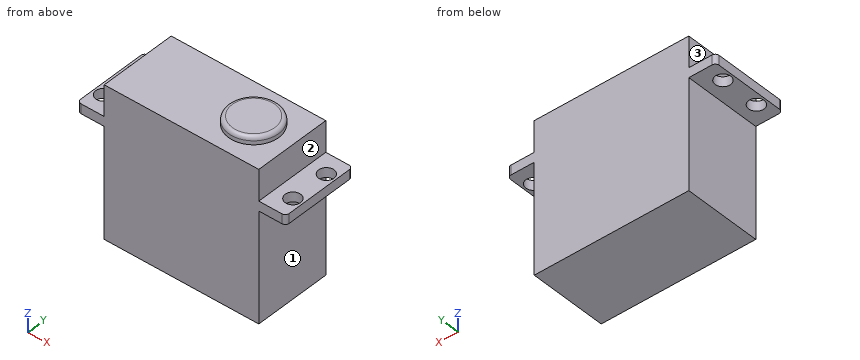
from build123d import *

# Parameters (mm, degrees)
PAD050_DEPTH    = 10
SKETCH087_R     = 2
POCKET033_DEPTH = 47.001
FILLET024_R     = 1
SKETCH235_R     = 6.5
PAD096_DEPTH    = 2
FILLET011_R     = 1


with BuildPart() as part:
    # Sketch086 → Pad050 (new body, symmetric)
    with BuildSketch(Plane.XZ):
        Polygon((-37, -18.5), (-37, -16), (-30, -16), (-30, -8), (10, -8), (10, -16), (17, -16), (17, -18.5), (10, -18.5), (10, -47), (-30, -47), (-30, -18.5), align=None)
    extrude(amount=PAD050_DEPTH, both=True)

    # Sketch087 → Pocket033 (cut, through all)
    with BuildSketch(Plane.XY):
        with Locations((14.5, 5)):
            Circle(SKETCH087_R)
        with Locations((14.5, -5)):
            Circle(SKETCH087_R)
        with Locations((-34.5, 5)):
            Circle(SKETCH087_R)
        with Locations((-34.5, -5)):
            Circle(SKETCH087_R)
    extrude(amount=-POCKET033_DEPTH, mode=Mode.SUBTRACT)

    # Fillet024
    fillet024_edges = [part.edges().sort_by_distance(p)[0] for p in [
        (17, -10, -17.25),
        (17, 10, -17.25),
        (-37, -10, -17.25),
        (-37, 10, -17.25),
    ]]
    fillet(fillet024_edges, radius=FILLET024_R)

    # Sketch235 (on Face12 of Fillet024) → Pad096 (join)
    with BuildSketch(Plane(origin=(0, 0, -8), x_dir=(-1, 0, 0), z_dir=(0, 0, 1))):
        Circle(SKETCH235_R)
    extrude(amount=PAD096_DEPTH)

    # Fillet011
    fillet011_edges = [part.edges().sort_by_distance(p)[0] for p in [
        (6.5, 0, -6),
    ]]
    fillet(fillet011_edges, radius=FILLET011_R)


with BuildPart() as part_1:
    # Body041 placement: moved
    add(part.part.moved(Location((0, 0, -1))))


solid = part_1.part
Part model, mm, in its own coordinate system. Face numbers are marked on the shaded views. A direction names the side the tool comes from. Coordinates: 2 decimals unless noted, no trailing zeros. Write each loop counter-clockwise with the first axis right and the second up, starting at its lowest first coordinate (ties: lowest second). Pieces come first, ordered by that corner, then holes. Notation, with made-up numbers: M 18,-32.5 L 54,-32.5 A24 cw 54,-8.5 Z; hole C 15.5,23 d9. An arc over 180 degrees is marked long. Return JSON: item names as keys, results as strings.
1. Flat gauge pins, fed straight in: pin 1 Ø7.5 at (x, y) = (-34.5, 0.5) entering from +Z; pin 2 Ø1 at (y, z) = (-7, -26) entering from +X; pin 3 Ø4 at (y, z) = (0.5, -11) entering from -X; pin 4 Ø2.5 at (x, y) = (-34.5, 5) entering from +Z. Where does each tip first touch, or does it go through?
Determined:
{"pin 1": "z = -17", "pin 2": "x = 10", "pin 3": "x = -30", "pin 4": "through"}
2. Saw through at B-B, the plane z = -18. Write the cut outline in (x, y).
Determined:
{"outline": "M -37,-9 A1 ccw -36,-10 L 16,-10 A1 ccw 17,-9 L 17,9 A1 ccw 16,10 L -36,10 A1 ccw -37,9 Z; hole C -34.5,-5 d4; hole C -34.5,5 d4; hole C 14.5,-5 d4; hole C 14.5,5 d4"}
3. Saw through at C-C, the plane y = 0. Write the cut outline in (x, z), then the cut area to 3 significant figures.
Determined:
{"outline": "M -37,-19.5 L -30,-19.5 L -30,-48 L 10,-48 L 10,-19.5 L 17,-19.5 L 17,-17 L 10,-17 L 10,-9 L 6.5,-9 L 6.5,-8 A1 ccw 5.5,-7 L -5.5,-7 A1 ccw -6.5,-8 L -6.5,-9 L -30,-9 L -30,-17 L -37,-17 Z", "area": "1,620 mm²"}
4. Saw through at D-D, the plane x = 0. Write the cut outline in (y, z), then the cut area to 3 significant figures.
Determined:
{"outline": "M -10,-48 L 10,-48 L 10,-9 L 6.5,-9 L 6.5,-8 A1 ccw 5.5,-7 L -5.5,-7 A1 ccw -6.5,-8 L -6.5,-9 L -10,-9 Z", "area": "806 mm²"}
5. Probe L1, parallel to Y at x = -34.5, z = -18.8; L2, parallel to Y at x = 14, z = -18; L3, parallel to X at y = 4, z = -19. List the from-to ranges inside material, lowest first.
Determined:
{"L1": "-10 to -7, -3 to 3, 7 to 10", "L2": "-10 to -6.94, -3.06 to 3.06, 6.94 to 10", "L3": "-37 to -36.23, -32.77 to 12.77, 16.23 to 17"}
6. Saw through at A-A, the plane x = -34.5. Write the cut outline in (y, z), then the cut area to 3 significant figures.
Determined:
{"outline": "M -10,-19.5 L -7,-19.5 L -7,-17 L -10,-17 Z; M -3,-19.5 L 3,-19.5 L 3,-17 L -3,-17 Z; M 7,-19.5 L 10,-19.5 L 10,-17 L 7,-17 Z", "area": "30.0 mm²"}
7. 3-axis set-ups, long thin cutter, end or side, ignore diameter. For the marked faces 1, 2 and 3: which of +Z, -Z, +X, -X, +Y, -Y reach the whole face in a straight line?
Determined:
{"face 1": "-Z, +X, +Y, -Y", "face 2": "+Z, +X, +Y, -Y", "face 3": "+Z, -X, +Y, -Y"}
